Here's how the part is built. I have some questions about the finished solid (model axes, mm). Round coordinates to 2 decimals unless told otherwise and drop trailing zeros. Order: outer loops, then holes, each group sorted by start corner. A loop starts at its lowest first (then second) coordinate and runs counter-clockwise, first axis right, second up. Notation, with made-up numbers: (33, -5.75) - (37, -5.75) arc R14 ccw to (37, -0.75) - close; hole circle Ø9 at (42, -34.5). An arc over 180 degrees is marked (long way). Answer as a JSON object with one key per item and string values.
```python
from build123d import *

# Parameters (mm, degrees)
F0_W     = 23
F0_H     = 50
F1_DEPTH = 15
F4_R     = 4.5
F5_DEPTH = 16
F6_W     = 23
F6_H     = 50
F7_DEPTH = 8


# Not quite as in the source:
# - a feature of the source that left no trace in its solid (it failed there, or was rolled back) is left out


with BuildPart() as f1:
    # F0 (on Top) → F1 (new body)
    with BuildSketch(Plane.XY):
        Rectangle(F0_W, F0_H)
    extrude(amount=-F1_DEPTH)

    # F4 (on face) → F5 (cut)
    with BuildSketch(Plane.XY):
        Circle(F4_R)
    extrude(amount=-F5_DEPTH, mode=Mode.SUBTRACT)

    # F6 (on face) → F7 (cut)
    with BuildSketch(Plane.XY):
        Rectangle(F6_W, F6_H)
    extrude(amount=-F7_DEPTH, mode=Mode.SUBTRACT)


solid = f1.part
```
1. Imagine slicing it at A-A (x = 0). List the corners of the cut face in (y, z) for me, plus the area to 3 significant figures.
Responses:
{"outline": "(-25, -15) - (-4.5, -15) - (-4.5, -8) - (-25, -8) - close; (4.5, -15) - (25, -15) - (25, -8) - (4.5, -8) - close", "area": "287 mm2"}
2. If I drill on L1, parallel to Y at x = 0, z = -10.5; L2, parallel to Y at x = 2.75, z = -10.75, over which ranges is the centre line in solid material (lowest first)? Write a range as [from, to].
Responses:
{"L1": "[-25, -4.5], [4.5, 25]", "L2": "[-25, -3.56], [3.56, 25]"}
3. Imagine slicing it at B-B (y = 0). List the corners of the cut face in (x, z) for me.
Responses:
{"outline": "(-11.5, -15) - (-4.5, -15) - (-4.5, -8) - (-11.5, -8) - close; (4.5, -15) - (11.5, -15) - (11.5, -8) - (4.5, -8) - close"}
4. Imagine slicing it at C-C (z = -12.5). List the corners of the cut face in (x, y) for me, plus the area to 3 significant figures.
Responses:
{"outline": "(-11.5, -25) - (11.5, -25) - (11.5, 25) - (-11.5, 25) - close; hole circle Ø9 at (0, 0)", "area": "1,090 mm2"}
5. Thinking about a two-plate mould opening in Y: for faces 1 (the face through (-11.5, 0, -11)), 2 (the face through (0, 25, -11)), 3 (the face through (0, -25, -11)), 4 (the face through (-0.59, 4.46, -11.45)), which applies, pulls with the +Y half, pulls with the -Y half, needs draft (parallel to the pull), parting line crosses it, or undercut?
Responses:
{"face 1": "needs draft", "face 2": "pulls with the +Y half", "face 3": "pulls with the -Y half", "face 4": "undercut"}
